```python
from build123d import *

# Parameters (mm, degrees)
F1_DEPTH = 8
F2_R     = 4


with BuildPart() as f1:
    # F0 (on Top) → F1 (new body)
    with BuildSketch(Plane.XY):
        Polygon((0, 1219), (0, 0), (507, 0), (507, 457), (200, 457), (200, 1219), align=None)
    extrude(amount=F1_DEPTH)

    # F2
    f2_edges = [f1.edges().sort_by_distance(p)[0] for p in [
        (0, 609.5, 0),
        (253.5, 0, 0),
        (507, 228.5, 0),
        (353.5, 457, 0),
        (200, 838, 0),
        (100, 1219, 0),
    ]]
    fillet(f2_edges, radius=F2_R)


solid = f1.part
```
Can you work these out from the model? Positions are in its coordinate system, mm. Round coordinates to 2 decimals unless told otherwise and drop trailing zeros. Loops run counter-clockwise (first coordinate to the right, second up) from the corner with the lowest first, then second, coordinate; pieces in that order, holes last. Notation, with made-up numbers: M -30.5,23.25 L -20.5,23.25 A10 cw -20.5,32.25 Z; hole C 33,43 d8. An arc over 180 degrees is marked long. Write item = value, one per line. Start each with the question number.
(1) I'm going to push flat-ended pins straight in: P1, Ø2, axis at x = 356, z = 6.5, coming from the +Y side; P2, Ø2, axis at y = 955, z = 5.5, coming from the +X side. Where does each tip first touch, or does it pass through?
(2) Suppose I cut it at B-B on x = 353. Write out the boundary of the cut face in (y, z), plus the area to 3 significant figures.
(3) I need wall thicknesses on line 1 along Y through (x, z) = (66, 2.75); line 2 along X through (y, z) = (507.5, 3.5); line 3 along Y through (x, z) = (466.5, 4). Which ranges of each line are inside material? Lowest first, please.
(4) Suppose I cut it at A-A on z = 6.5. Write out the boundary of the cut face in (x, y), plus the area to 3 significant figures.
Answer block:
q1.P1 = 457
q1.P2 = 200
q2.outline = M 0,4 A4 ccw 4,0 L 453,0 A4 ccw 457,4 L 457,8 L 0,8 Z
q2.area = 3,650 mm²
q3.line_1 = 0.2 to 1218.8
q3.line_2 = 0.03 to 199.97
q3.line_3 = 0 to 457
q4.outline = M 0,0 L 507,0 L 507,457 L 200,457 L 200,1219 L 0,1219 Z
q4.area = 384,000 mm²
